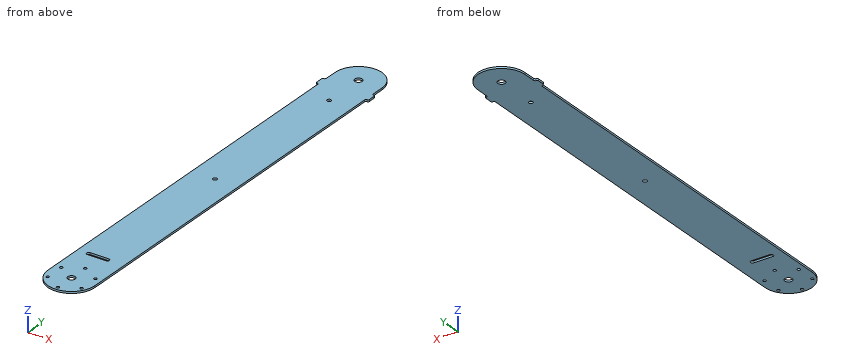
Autodesk Inventor part; units mm, degrees
ref_plane "YZ Plane" through (0, 0, 0) normal (1, 0, 0) x (0, 1, 0)
ref_plane "XZ Plane" through (0, 0, 0) normal (0, 1, 0) x (-1, 0, 0)
ref_plane "XY Plane" through (0, 0, 0) normal (0, 0, 1) x (1, 0, 0)
sketch "スケッチ1" plane through (0, 0, 0) normal (0, 0, 1) x (1, 0, 0)
  circle A0 centre (0, 0) radius 25
  circle A1 centre (0, 440) radius 25
  line L0 (-25, 0) -> (-25, 440)
  line L1 (25, 440) -> (25, 0)
  dimension "d0" = 50
  dimension "d1" = 50
  dimension "d2" = 440
extrude "プレート1" add sketch "スケッチ1" along normal blind 2
sketch "スケッチ4" plane through (0, 0, 0) normal (0, 0, -1) x (-1, 0, 0)
  circle A0 centre (0, 0) radius 4
  dimension "d28" = 8
extrude "押し出し1" cut sketch "スケッチ4" against normal blind 10
sketch "スケッチ5" plane through (0, 0, 0) normal (0, 0, -1) x (-1, 0, 0)
  circle A0 centre (0, 0) radius 21
  point P0 (0, 21)
  point P1 (-18.1865, 10.5)
  point P2 (-18.1865, -10.5)
  point P3 (0, -21)
  point P4 (18.1865, -10.5)
  point P5 (18.1865, 10.5)
  dimension "d31" = 42
  dimension "d34" = 360
hole "穴3" at (0, 21, 0) at (18.1865, 10.5, 0) at (18.1865, -10.5, 0) at (0, -21, 0) at (-18.1865, -10.5, 0) at (-18.1865, 10.5, 0) direction (0, 0, 1) diameter 3.2 end through all
sketch "スケッチ6" plane through (0, 0, 2) normal (0, 0, 1) x (1, 0, 0)
  arc A0 (25, 440) -> (-25, 440) centre (0, 440) ccw
  circle A1 centre (0, 440) radius 4
  point P0 (0, 0)
  dimension "d43" = 8
extrude "押し出し2" cut sketch "スケッチ6" against normal blind 10
sketch "スケッチ8" plane through (0, 0, 2) normal (0, 0, 1) x (1, 0, 0)
  arc A0 (25, 440) -> (-25, 440) centre (0, 440) ccw
  point P0 (0, 0)
  point P1 (-13, 45)
  point P2 (0, 395)
  point P3 (0, 220)
  dimension "d54" = 45
  dimension "d55" = 220
  dimension "d71" = 45
  dimension "d72" = 13
hole "穴4" at (-13, 45, 2) at (0, 395, 2) at (0, 220, 2) direction (0, 0, -1) diameter 4.3 end through all
sketch "スケッチ10" plane through (0, 0, 2) normal (0, 0, 1) x (1, 0, 0)
  circle A0 centre (7, 45) radius 2.15
  line L0 (7, 45) -> (-13, 45) construction
  line L1 (7, 47.15) -> (-13, 47.15)
  line L2 (-13, 42.85) -> (7, 42.85)
  arc A1 (7, 42.85) -> (7, 47.15) centre (7, 45) ccw
  arc A2 (-13, 47.15) -> (-13, 42.85) centre (-13, 45) ccw
  circle A3 centre (-13, 45) radius 2.15
  point P0 (0, 0)
  point P1 (-3, 45)
  point P2 (7, 47.15)
  point P3 (7, 42.85)
  dimension "d68" = 20
extrude "押し出し3" cut sketch "スケッチ10" against normal blind 10
sketch "スケッチ11" plane through (0, 0, 2) normal (0, 0, 1) x (1, 0, 0)
  circle A0 centre (25, 420) radius 3
  line L0 (25, 440) -> (25, 0)
  circle A1 centre (0, 440) radius 4
  line L1 (22, 425) -> (28, 425)
  line L2 (28, 425) -> (28, 415)
  line L3 (28, 415) -> (22, 415)
  line L4 (22, 415) -> (22, 425)
  line L5 (22, 425) -> (28, 415) construction
  line L6 (28, 425) -> (22, 415) construction
  point P0 (0, 0)
  point P1 (25, 423)
  point P2 (25, 417)
  point P3 (28, 420)
  dimension "d73" = 6
  dimension "d74" = 0
  dimension "d75" = 20
  dimension "d79" = 10
extrude "押し出し4" add sketch "スケッチ11" against normal up to surface (2 mm away) contours A0 L0 | L2 L3 L0 A0 | A0 L0 L1 L2 | L0 A0 | A0 L4 L1 L0 | L0 L3 L4 A0
fillet "コーナーR1" radius 1.5 4 edges at (25, 425, 1) (28, 425, 1) (28, 415, 1) (25, 415, 1)
mirror "ミラー1" about plane through (0, 0, 0) normal (1, 0, 0) of "押し出し4", "コーナーR1"
fillet_without_effect "コーナーR2"
equation "\"d41\" = Thickness"
equation "\"d3\" = Thickness"
equation "\"BendRadius\" = Thickness"
equation "\"BendReliefWidth\" = Thickness"
equation "\"BendReliefDepth\" = 0.5 * Thickness"
equation "\"CornerReliefSize\" = 4 * Thickness"
equation "\"MinimumRemnant\" = 2 * Thickness"
equation "\"TransitionRadius\" = BendRadius"
equation "\"JacobiRadiusSize\" = Thickness"
equation "\"GapSize\" = Thickness"
properties part number "link3-plate1" material "CFRP"
Design review of the part built by this model. Coordinates are the model's own, in mm. Coordinates: 2 decimals unless noted, no trailing zeros. Loops run counter-clockwise (first coordinate to the right, second up) from the corner with the lowest first, then second, coordinate; pieces in that order, holes last. Notation, with made-up numbers: (9.5, -19) - (23.5, -19) arc R28 ccw to (23.5, 7) - close; hole circle Ø1 at (68, 63.25). An arc over 180 degrees is marked (long way). Use CSV: the item, a comma, the result in double quotes. Start each with the question number.
1. Add section A-A on z = 0.85. Count the separate pieces of the cut face and the enclosed holes in it, plus the area to 3 significant figures.
2. Add section B-B on x = -9. Give the boundary of the cut face in (y, z).
3. Add section C-C on y = 266. Give the boundary of the cut face in (x, z).
4. To check wall thickness, follow probe 1 along Y at (x, z) = (-19.5, 1.85); probe 2 along X at (y, z) = (414, 0.6); probe 3 along Y at (x, z) = (17.5, 1.2). State the ranges of each line that lie inside material, in increasing order.
5. Clearance check with flat-ended pins moving along their axes: pin 1 (0.6 mm diameter, centred on y = 434, z = 1, fed in from -X); pin 2 (0.6 mm diameter, centred on x = -4, z = 0.5, fed in from -Y). State where each tip first meets the part, or that it passes through.
Resolved:
1,separate pieces,"1"
1,enclosed holes,"11"
1,area,"23,700 mm2"
2,outline,"(-23.32, 0) - (42.85, 0) - (42.85, 2) - (-23.32, 2) - close; (47.15, 0) - (463.32, 0) - (463.32, 2) - (47.15, 2) - close"
3,outline,"(-25, 0) - (25, 0) - (25, 2) - (-25, 2) - close"
4,probe 1,"-15.64 to -11.41, -9.59 to 9.59, 11.41 to 455.64"
4,probe 2,"-25.09 to 25.09"
4,probe 3,"-17.85 to -11.95, -9.05 to 9.05, 11.95 to 457.85"
5,pin 1,"x = -25"
5,pin 2,"y = -24.72"
